Autodesk Inventor part; units mm, degrees
ref_plane "YZ Plane" through (0, 0, 0) normal (1, 0, 0) x (0, 1, 0)
ref_plane "XZ Plane" through (0, 0, 0) normal (0, 1, 0) x (-1, 0, 0)
ref_plane "XY Plane" through (0, 0, 0) normal (0, 0, 1) x (1, 0, 0)
sketch "Эскиз1" plane through (0, 0, 0) normal (0, 1, 0) x (-1, 0, 0)
  line L0 (-4.0164, 1.5133) -> (-8.1434, 1.5133)
  circle A0 centre (-6.6434, 0.0133) radius 0.75
  line L1 (-4.0164, -1.4867) -> (-8.1434, -1.4867)
  line L2 (-4.0164, 1.5133) -> (-4.0164, -1.4867)
  line L3 (-4.0164, 1.5133) -> (-8.1434, 1.5133)
  line L4 (-8.1434, 1.5133) -> (-8.1434, -1.4867)
  circle A1 centre (6.3566, 0.0133) radius 0.75
  line L5 (3.7295, -1.4867) -> (3.7295, 1.5133)
  line L6 (7.8566, -1.4867) -> (3.7295, -1.4867)
  line L7 (7.8566, 1.5133) -> (7.8566, -1.4867)
  line L8 (3.7295, 1.5133) -> (7.8566, 1.5133)
  line L9 (-4.0164, 1.5133) -> (-4.0164, -1.4867)
  line L10 (3.7295, -1.4867) -> (-4.0164, -1.4867)
  line L11 (3.7295, -1.4867) -> (3.7295, 1.5133)
  line L12 (-4.0164, 1.5133) -> (3.7295, 1.5133)
  point P0 (0, 0)
  point P1 (0, 0)
extrude "Выдавливание1" add sketch "Эскиз1" along normal blind 5
sketch "Эскиз2" plane through (-7.8566, 0, 1.5133) normal (0, 0, 1) x (1, 0, 0)
  circle A0 centre (8, -0.857) radius 4
  line L0 (0, 0) -> (16, 0)
  dimension "d2" = 8
  dimension "d6" = 0.857
  dimension "d7" = 8
extrude "Выдавливание2" cut sketch "Эскиз2" against normal through all
properties part number "КВ33.044.208 - Зажим вакумной присоски"
Work out the finished part from the listing and answer in its coordinate system (mm). Give positions to 0.01 mm unless a question says otherwise; leave off trailing zeros. Write each loop counter-clockwise with the first axis right and the second up, starting at its lowest first coordinate (ties: lowest second). Pieces come first, ordered by that corner, then holes. Notation, with made-up numbers: (65, -4) - (76, -4) arc R8 cw to (76, 0) - close; hole circle Ø3 at (17.5, -4). An arc over 180 degrees is marked (long way). One line per item, written item: value. Start each with the question number.
1. Find section A-A (y = 2.2). Write down the section's boundary in (x, z).
2. Find section B-B (z = 0.45). Write down the section's boundary in (x, y), then the cut area to 3 significant figures.
3. For a pull along Z with two mould halves and no side action, classify faces 1 (the cylindrical face through (5.95, 2.46, 0.3)), 2 (the flat face through (0, 4, 1.513)), 3 (the flat face through (8.143, 2, 0)) as +Z half, -Z half, draft (parallel to the pull), parting line (faces both ways), or undercut.
4. Consider probe 1 along X at (y, z) = (4.1, -0.05); probe 2 along X at (y, z) = (1.75, -0.5); probe 3 along X at (y, z) = (2.65, 0.65). Determine where each line is inside the solid, lowest interval first.
5. Find section C-C (x = -6.75). Write down the section's boundary in (y, z), then the cut area to 3 significant figures.
6. Find section D-D (z = 1.15). Write down the section's boundary in (x, y), then the cut area to 3 significant figures.
7. Given pin 1 (1.5 mm diameter, centred on x = -2.5, z = 1, fed in from -Y); pin 2 (1 mm diameter, centred on x = -2, y = 2, fed in from +Z), each flat-ended and moving along its own axis, determine where each tip first touches the part or whether it passes through.
Geometry results:
1. outline: (-7.86, -1.49) - (-2.44, -1.49) - (-2.44, 1.51) - (-7.86, 1.51) - close; (2.72, -1.49) - (8.14, -1.49) - (8.14, 1.51) - (2.72, 1.51) - close; hole circle Ø1.5 at (-6.36, 0.01); hole circle Ø1.5 at (6.64, 0.01)
2. outline: (-7.86, 0) - (-6.97, 0) - (-6.97, 5) - (-7.86, 5) - close; (-5.75, 0) - (-3.76, 0) arc R4 cw to (4.05, 0) - (6.03, 0) - (6.03, 5) - (-5.75, 5) - close; (7.25, 0) - (8.14, 0) - (8.14, 5) - (7.25, 5) - close
2. area: 49.5 mm2
3. face 1: undercut
3. face 2: +Z half
3. face 3: draft
4. probe 1: -7.86 to -7.1, -5.61 to 5.9, 7.39 to 8.14
4. probe 2: -7.86 to -6.9, -5.81 to -2.89, 3.18 to 6.1, 7.19 to 8.14
4. probe 3: -7.86 to -6.75, -5.96 to -1.78, 2.07 to 6.25, 7.04 to 8.14
5. outline: (0, -1.49) - (5, -1.49) - (5, -0.63) - (0, -0.63) - close; (0, 0.65) - (5, 0.65) - (5, 1.51) - (0, 1.51) - close
5. area: 8.61 mm2
6. outline: (-7.86, 0) - (-3.76, 0) arc R4 cw to (4.05, 0) - (8.14, 0) - (8.14, 5) - (-7.86, 5) - close
6. area: 61.7 mm2
7. pin 1: y = 1.26
7. pin 2: z = 1.51
